Build history of the part. All positions in model axes, mm. Give positions to 0.01 mm unless a question says otherwise; leave off trailing zeros. Loops run counter-clockwise (first coordinate to the right, second up) from the corner with the lowest first, then second, coordinate; pieces in that order, holes last. Notation, with made-up numbers: M 37.25,-10 L 55.25,-10 A26 cw 55.25,6 Z; hole C 27.5,-27 d8. An arc over 180 degrees is marked long. Answer as a JSON object with one key per item and string values. Group by question number.
1. Drill centre lines: line 1 along X through (y, z) = (4.5, 13.5); line 2 along Y through (x, z) = (-19, -3.5); line 3 along Y through (x, z) = (0.5, 21). Where is each one in solid material? Low to high. Write a range as [from, to].
2. Slice it at B-B (z = 11.5). List the corners of the cut face in (x, y), then the cut area to 3 significant figures.
3. Drop flat-ended pins along their axis: pin 1 Ø0.5 at (x, y) = (-18.5, 4.5) entering from -Z; pin 2 Ø6 at (x, y) = (-17, 10) entering from -Z; pin 3 Ø4.5 at (x, z) = (17, 5) entering from +Y; pin 4 Ø1.5 at (x, y) = (5.5, 4) entering from -Z. Give the stop position or say it passes through.
4. Slice it at A-A (x = -18.5). List the corners of the cut face in (y, z).
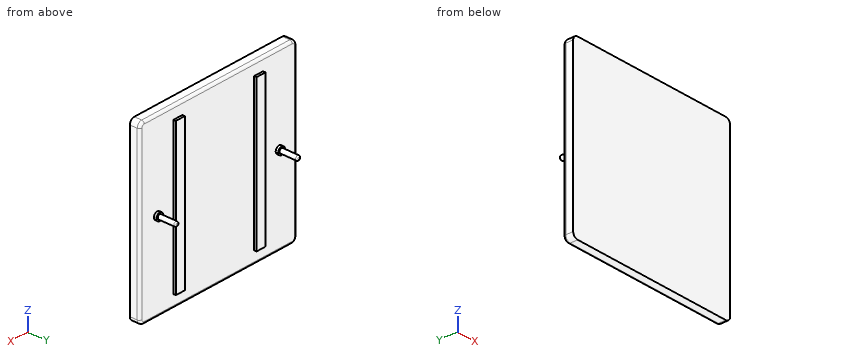
Autodesk Inventor part; units mm, degrees
ref_plane "YZ Plane" through (0, 0, 0) normal (1, 0, 0) x (0, 1, 0)
ref_plane "XZ Plane" through (0, 0, 0) normal (0, 1, 0) x (-1, 0, 0)
ref_plane "XY Plane" through (0, 0, 0) normal (0, 0, 1) x (1, 0, 0)
sketch "Sketch1" plane through (0, 0, 0) normal (0, 1, 0) x (-1, 0, 0)
  line L0 (-35, -35) -> (35, -35)
  line L1 (35, -35) -> (35, 35)
  line L2 (35, 35) -> (-35, 35)
  line L3 (-35, 35) -> (-35, -35)
  line L4 (-35, -35) -> (35, 35) construction
  line L5 (35, -35) -> (-35, 35) construction
  point P0 (0, 0)
  dimension "d0" = 70
  dimension "d1" = 70
extrude "Extrusion1" add sketch "Sketch1" along normal blind 4
sketch "Sketch2" plane through (0, 4, 0) normal (0, 1, 0) x (1, 0, 0)
  circle A0 centre (-27.15, 0) radius 0.9
  circle A1 centre (27.15, 0) radius 0.9
  point P0 (0, 0)
  dimension "d4" = 1.8
  dimension "d5" = 1.8
  dimension "d6" = 54.3
  dimension "d7" = 27.15
extrude "Extrusion2" add sketch "Sketch2" along normal blind 8
fillet "Fillet1" radius 2 4 edges at (35, 2, 35) (-35, 2, 35) (-35, 2, -35) (35, 2, -35)
fillet "Fillet2" radius 0.5 2 edges at (26.25, 12, 0) (-28.05, 12, 0)
sketch "Sketch3" plane through (0, 4, 0) normal (0, 1, 0) x (1, 0, 0)
  circle A0 centre (27.15, 0) radius 0.9
  circle A1 centre (27.15, 0) radius 1.5
  circle A2 centre (-27.15, 0) radius 0.9
  circle A3 centre (-27.15, 0) radius 1.5
  line L0 (-16, -30) -> (-20, -30)
  line L1 (-20, -30) -> (-20, 30)
  line L2 (-20, 30) -> (-16, 30)
  line L3 (-16, 30) -> (-16, -30)
  line L4 (-16, -30) -> (-20, 30) construction
  line L5 (-20, -30) -> (-16, 30) construction
  line L6 (20, -30) -> (16, -30)
  line L7 (16, -30) -> (16, 30)
  line L8 (16, 30) -> (20, 30)
  line L9 (20, 30) -> (20, -30)
  line L10 (20, -30) -> (16, 30) construction
  line L11 (16, -30) -> (20, 30) construction
  point P0 (0, 0)
  point P1 (-18, 0)
  point P2 (18, 0)
  dimension "d12" = 18
  dimension "d13" = 60
  dimension "d14" = 60
  dimension "d15" = 18
  dimension "d16" = 4
  dimension "d17" = 4
  dimension "d18" = 3
  dimension "d19" = 3
extrude "Extrusion3" add sketch "Sketch3" along normal blind 1 contours A0 | A1 | A2 | A3 | L0 L1 L2 L3 | L6 L7 L8 L9
fillet "Fillet3" radius 1 8 edges at (34.4142, 4, 34.4142) (35, 4, 0) (34.4142, 4, -34.4142) (0, 4, -35) (-34.4142, 4, -34.4142) (-35, 4, 0) (-34.4142, 4, 34.4142) (0, 4, 35)
equation "\"d5\" = d4"
equation "\"d14\" = d13"
equation "\"d17\" = d16"
equation "\"d19\" = d18"
properties part number "Installation Base"
Established:
{
 "1": {"line 1": "x = [-20, -16], [16, 20]", "line 2": "y = [0, 5]", "line 3": "y = [0, 4]"},
 "2": {"outline": "M -35,0 L 35,0 L 35,3 A1 ccw 34,4 L 20,4 L 20,5 L 16,5 L 16,4 L -16,4 L -16,5 L -20,5 L -20,4 L -34,4 A1 ccw -35,3 Z", "area": "288 mm^2"},
 "3": {"pin 1": "stops at z = -30", "pin 2": "passes through", "pin 3": "stops at y = 5", "pin 4": "stops at z = -34.97"},
 "4": {"outline": "M 0,-35 L 3,-35 A1 ccw 4,-34 L 4,-30 L 5,-30 L 5,30 L 4,30 L 4,34 A1 ccw 3,35 L 0,35 Z"}
}
